Autodesk Inventor part; units mm, degrees
ref_plane "Work Plane1" through (0, 0, 5) normal (0, 0, -1) x (-1, 0, 0)
ref_plane "YZ Plane" through (0, 0, 0) normal (1, 0, 0) x (0, 1, 0)
ref_plane "XZ Plane" through (0, 0, 0) normal (0, 1, 0) x (-1, 0, 0)
sketch "Sketch4" plane through (0, 0, 0) normal (1, 0, 0) x (0, 1, 0)
  circle A0 centre (0, 0) radius 27.5
  circle A1 centre (0, 0) radius 26
  line L0 (0, 0) -> (0, 27.5)
  line L1 (0, 27.5) -> (5.5, 27.5)
  line L2 (5.5, 27.5) -> (5.5, 25.4116)
  line L3 (0, 27.5) -> (-5.5, 27.5)
  line L4 (-5.5, 27.5) -> (-5.5, 25.4116)
  line L5 (27.5, 0) -> (-27.5, 0)
  point P0 (26, 0)
  point P1 (5.5, 26.9444)
  dimension "d20" = 55
  dimension "d21" = 52
  dimension "d22" = 5.5
  dimension "d23" = 5.5
revolve "Revolution2" add sketch "Sketch4" angle 360 about axis through (0, 0, 0) along (0, 0, 1) contours L5 A1 L2 A0
ref_plane "Work Plane1" through (0, 0, 5) normal (0, 0, -1) x (-1, 0, 0)
sketch "Sketch5" plane through (0, 0, 5) normal (0, 0, -1) x (-1, 0, 0)
  line L0 (-12, -12.25) -> (12, -12.25)
  line L1 (12, -12.25) -> (12, 12.25)
  line L2 (12, 12.25) -> (-12, 12.25)
  line L3 (-12, 12.25) -> (-12, -12.25)
  line L4 (-12, -12.25) -> (12, 12.25) construction
  line L5 (12, -12.25) -> (-12, 12.25) construction
  circle A0 centre (-12, 12.25) radius 1.25
  circle A1 centre (12, 12.25) radius 1.25
  circle A2 centre (12, -12.25) radius 1.25
  circle A3 centre (-12, -12.25) radius 1.25
  point P0 (0, 0)
  dimension "d26" = 24
  dimension "d27" = 24.5
  dimension "d28" = 2.5
extrude "Extrusion3" add sketch "Sketch5" against normal up to surface contours L3 A3 L0 | L0 A3 L3 | A2 L1 L0 | L0 L1 A2 | A0 L2 L3 | L3 L2 A0 | A1 L2 L1 | L1 L2 A1
sketch "Sketch6" plane through (0, 0, 0) normal (0, 0, -1) x (-1, 0, 0)
  circle A0 centre (0, 0) radius 26
  line L0 (-26, 0) -> (-26.75, 0)
  line L1 (-26.75, 0) -> (-26.75, 3)
  line L2 (-26.75, 3) -> (26.75, 3)
  line L3 (26.75, 3) -> (26.75, -3)
  line L4 (26.75, -3) -> (-26.75, -3)
  line L5 (-26.75, -3) -> (-26.75, 3)
  line L6 (0, 26) -> (0, 26.75)
  line L7 (0, 26.75) -> (3, 26.75)
  line L8 (3, 26.75) -> (-3, 26.75)
  line L9 (-3, 26.75) -> (-3, -26.75)
  line L10 (-3, -26.75) -> (3, -26.75)
  line L11 (3, -26.75) -> (3, 26.75)
  point P0 (-3, 3)
  point P1 (-25.8263, 3)
  point P2 (-25.8263, -3)
  point P3 (25.8263, -3)
  point P4 (25.8263, 3)
  point P5 (3, 3)
  point P6 (3, 25.8263)
  point P7 (-3, 25.8263)
  point P8 (3, -25.8263)
  point P9 (-3, -25.8263)
  point P10 (3, -3)
  point P11 (-3, -3)
  dimension "d31" = 0.75
  dimension "d32" = 3
  dimension "d33" = 53.5
  dimension "d34" = 6
  dimension "d35" = 0.75
  dimension "d36" = 3
  dimension "d37" = 6
  dimension "d38" = 53.5
extrude "Extrusion4" add sketch "Sketch6" against normal blind 3 contours A0 L4 L11 L2 | L11 L2 L9 A0 | L11 L4 L9 L2 | L9 L4 A0 L2
sketch "Sketch7" plane through (0, 0, 0) normal (0, 0, -1) x (-1, 0, 0)
  line L0 (0, 0) -> (22.5, 0)
  line L1 (0, 0) -> (-22.5, 0)
  line L2 (0, 0) -> (0, 22.5)
  circle A0 centre (0, 22.5) radius 1.6
  circle A1 centre (-22.5, 0) radius 1.6
  circle A2 centre (22.5, 0) radius 1.6
  dimension "d41" = 22.5
  dimension "d42" = 22.5
  dimension "d43" = 22.5
  dimension "d44" = 3.2
  dimension "d45" = 3.2
  dimension "d46" = 3.2
extrude "Extrusion5" cut sketch "Sketch7" against normal up to surface
sketch "Sketch8" plane through (0, 0, 0) normal (0, 0, -1) x (-1, 0, 0)
  circle A0 centre (0, 0) radius 2.5
  circle A1 centre (0, 0) radius 2
  line L0 (2.5, -0.7) -> (-2.5, -0.7)
  line L1 (-2.5, -0.7) -> (-2.5, 0.7)
  line L2 (-2.5, 0.7) -> (2.5, 0.7)
  line L3 (2.5, 0.7) -> (2.5, -0.7)
  line L4 (2.5, -0.7) -> (-2.5, 0.7) construction
  line L5 (-2.5, -0.7) -> (2.5, 0.7) construction
  line L6 (-0.7, -2.5) -> (-0.7, 2.5)
  line L7 (-0.7, 2.5) -> (0.7, 2.5)
  line L8 (0.7, 2.5) -> (0.7, -2.5)
  line L9 (0.7, -2.5) -> (-0.7, -2.5)
  line L10 (-0.7, -2.5) -> (0.7, 2.5) construction
  line L11 (-0.7, 2.5) -> (0.7, -2.5) construction
  point P0 (-0.7, 1.8735)
  point P1 (-1.8735, 0.7)
  point P2 (-2.4, 0.7)
  point P3 (-2.4, -0.7)
  point P4 (-1.8735, -0.7)
  point P5 (-0.7, -1.8735)
  point P6 (-0.7, -2.4)
  point P7 (0.7, -2.4)
  point P8 (0.7, -1.8735)
  point P9 (1.8735, -0.7)
  point P10 (2.4, -0.7)
  point P11 (2.4, 0.7)
  point P12 (1.8735, 0.7)
  point P13 (0.7, 1.8735)
  point P14 (0.7, 2.4)
  point P15 (-0.7, 2.4)
  dimension "d49" = 5
  dimension "d50" = 4
  dimension "d51" = 1.4
  dimension "d52" = 1.4
extrude "Extrusion6" cut sketch "Sketch8" against normal blind 10 contours A0 L0 A1 L2 | L8 A1 L6 A0 | L2 L8 A1 | A1 L0 L8 L2 | A0 L6 A1 L8 | A1 L8 L0 | L8 L2 L6 A1 | L8 L0 L6 L2 | A1 L6 L0 L8 | L6 L2 A1 | L6 L0 A1 L2 | A1 L0 L6 | L2 A1 L0 A0
equation "\"d39\" = d32"
properties part number "Eye"
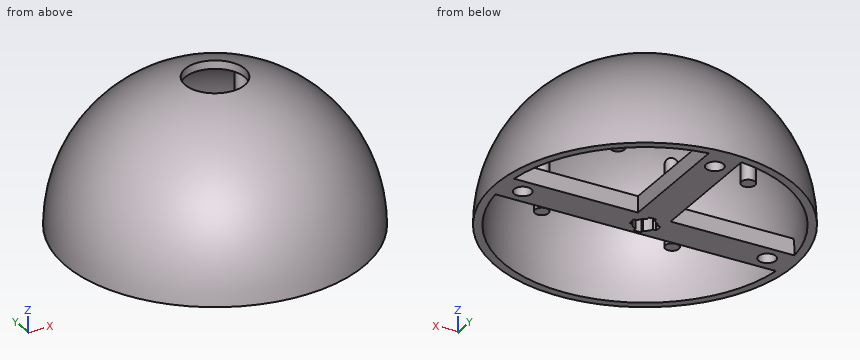
The listing builds one solid part. Answer for the finished solid, in the listing's coordinates (mm). Round coordinates to 2 decimals unless told otherwise and drop trailing zeros. Write each loop counter-clockwise with the first axis right and the second up, starting at its lowest first coordinate (ties: lowest second). Pieces come first, ordered by that corner, then holes. Notation, with made-up numbers: (17, 75) -> (71, 75) arc R32 ccw to (71, 105) -> close; hole circle Ø7 at (34, 82). An arc over 180 degrees is marked (long way). Answer as a JSON object with one key per item and string values. Group by question number.
Q1. Section C-C (y = 22.5) is taken. Write down the section's boundary in (x, z), plus the area to 3 significant figures.
Q2. Each of these flat-tipped pins is pushed along its axis until it touches: pin 1 Ø0.9 at (y, z) = (17.5, 1.5) entering from +X; pin 2 Ø3.5 at (x, z) = (-19, 1) entering from +Y; pin 3 Ø0.6 at (y, z) = (2, 1) entering from +X. Where does it stop, or does it pass through?
Q3. Section A-A (x = 0) is taken. Write down the section's boundary in (y, z).
Q4. Section D-D (x = -12) is taken. Write down the section's boundary in (y, z), plus the area to 3 significant figures.
Q5. Section B-B (z = 8) is taken. Write down the section's boundary in (x, y).
Q6. Straight lines are drawn through the part: line 1 along Y through (x, z) = (0, 2.2); line 2 along Y through (x, z) = (0, 1.05); line 3 along X through (y, z) = (12, 4.25). For each, find the intervals that lie inside material, in ascending order.
Check values:
{
 "1": {"outline": "(-15.81, 0) -> (-13.03, 0) arc R13.03 cw to (13.03, 0) -> (15.81, 0) arc R15.81 ccw to start; (-3, 0) -> (-1.6, 0) -> (-1.6, 3) -> (-3, 3) -> close; (1.6, 0) -> (3, 0) -> (3, 3) -> (1.6, 3) -> close", "area": "134 mm^2"},
 "2": {"pin 1": "x = 21.53", "pin 2": "y = 21.4", "pin 3": "x = 27.43"},
 "3": {"outline": "(-27.5, 0) -> (-26, 0) arc R26 cw to (-5.5, 25.41) -> (-5.5, 26.94) arc R27.5 ccw to start; (-3, 0) -> (-2.5, 0) -> (-2.5, 3) -> (-3, 3) -> close; (2.5, 0) -> (20.9, 0) -> (20.9, 3) -> (2.5, 3) -> close; (5.5, 25.41) arc R26 cw to (25.83, 3) -> (24.1, 3) -> (24.1, 0) -> (27.5, 0) arc R27.5 ccw to (5.5, 26.94) -> close"},
 "4": {"outline": "(-24.74, 0) -> (-23.07, 0) arc R23.07 cw to (-13.5, 18.7) -> (-13.5, 5) -> (-11, 5) -> (-11, 20.27) arc R23.07 cw to (11, 20.27) -> (11, 5) -> (13.5, 5) -> (13.5, 18.7) arc R23.07 cw to (23.07, 0) -> (24.74, 0) arc R24.74 ccw to start; (-3, 0) -> (3, 0) -> (3, 3) -> (-3, 3) -> close", "area": "217 mm^2"},
 "5": {"outline": "circle Ø52.62 at (0, 0); circle Ø2.5 at (-12, -12.25); circle Ø2.5 at (-12, 12.25); circle Ø2.5 at (12, -12.25); circle Ø2.5 at (12, 12.25); hole circle Ø49.48 at (0, 0)"},
 "6": {"line 1": "-27.41 to -25.91, -3 to -2.5, 2.5 to 20.9, 24.1 to 27.41", "line 2": "-27.48 to -25.98, -3 to -2.5, 2.5 to 20.9, 24.1 to 27.48", "line 3": "-24.38 to -22.67, 22.67 to 24.38"}
}
